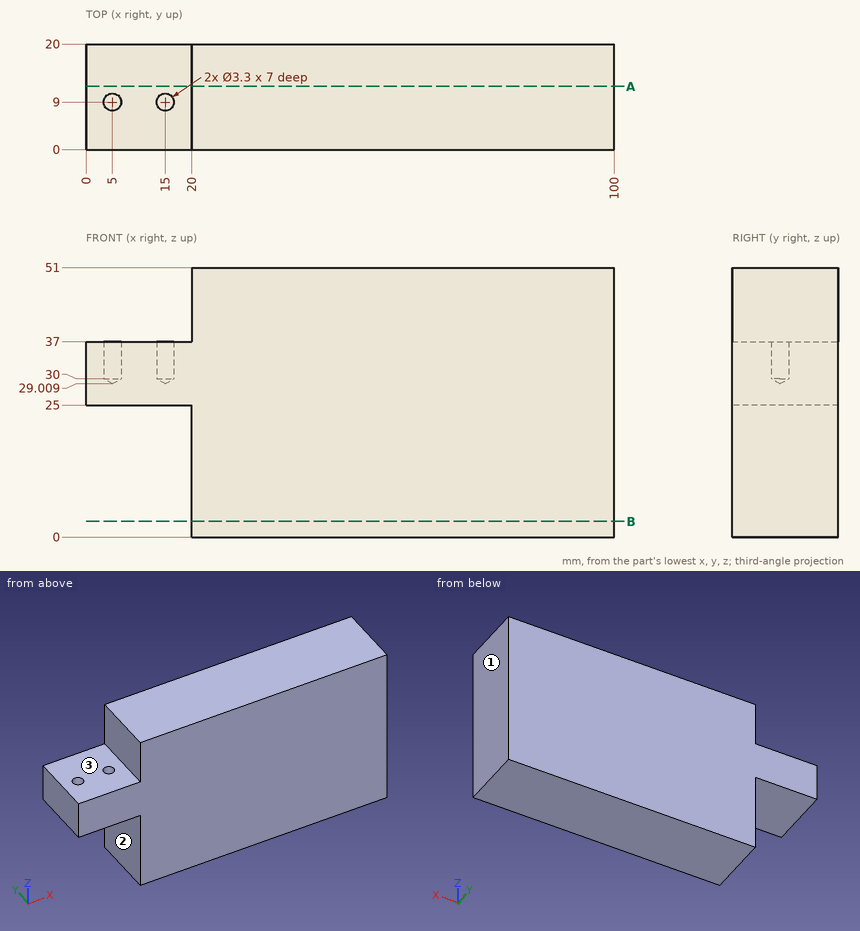
Print and shaded views of the part. All mm, measured from the part's lowest x, y and z. A direction names the side the tool comes from. Give positions to 0.01 mm unless a question says otherwise; leave off trailing zeros. Write each loop counter-clockwise with the first axis right and the second up, starting at its lowest first coordinate (ties: lowest second). Pieces come first, ordered by that corner, then holes. Notation, with made-up numbers: (25.5, 65.5) - (35.5, 65.5) arc R25 ccw to (35.5, 96.5) - close; hole circle Ø11 at (15, -32.5). An arc over 180 degrees is marked (long way). One line per question, with ' | ' between items. Start each with the question number.
(1) Slice it at B-B on z = 3. Write the cut outline in (x, y), plus the area to 3 significant figures.
(2) Pin check, flat tips, straight feed: P1, Ø6, axis at x = 14, y = 13.5, coming from the -Z side; P2, Ø10, axis at y = 9, z = 9.5, coming from the -X side; P3, Ø4.5, axis at x = 15, y = 9, coming from the +Z side. Stop position of each tip, or through.
(3) Wall check: line 1 along X through (y, z) = (9, 32); line 2 along Y through (x, z) = (5, 34.25); line 3 along Z through (x, y) = (18.5, 7.25). Give the ranges that are in metal, low to high. Write a range as from..to.
(4) 3-axis set-ups, long thin cutter, end or side, ignore diameter. For the marked faces 1, 2 and 3: which of +Z, -Z, +X, -X, +Y, -Y reach the whole face in a straight line?
(5) Slice it at A-A on y = 12. Write the cut outline in (x, z), plus the area to 3 significant figures.
Results below:
1) outline: (20, 0) - (100, 0) - (100, 20) - (20, 20) - close | area: 1,600 mm^2
2) P1: z = 25 | P2: x = 20 | P3: z = 37
3) line 1: 0..3.35, 6.65..13.35, 16.65..100 | line 2: 0..7.35, 10.65..20 | line 3: 25..37
4) face 1: +Z, -Z, +X, +Y, -Y | face 2: -Z, -X, +Y, -Y | face 3: +Z, -X, +Y, -Y
5) outline: (0, 25) - (20, 25) - (20, 0) - (100, 0) - (100, 51) - (20, 51) - (20, 37) - (0, 37) - close | area: 4,320 mm^2
